Here's how the part is built. I have some questions about the finished solid (model axes, mm). A direction names the side the tool comes from. Round coordinates to 2 decimals unless told otherwise and drop trailing zeros. Loops run counter-clockwise (first coordinate to the right, second up) from the corner with the lowest first, then second, coordinate; pieces in that order, holes last. Notation, with made-up numbers: (26, 33) - (53, 33) arc R10 ccw to (53, 45) - close; hole circle Ø2 at (-8.5, 12.5). An arc over 180 degrees is marked (long way). Answer as a JSON object with one key per item and string values. Group by question number.
1) I want a section at A-A, the plane z = 0.75. Give the number of separate pieces and of enclosed holes in the cut face, then the cut area to 3 significant figures.
2) Will these pins go through, and if not, where does the flat tip stop? P1, Ø1.5, axis at x = 6, y = -3.5, coming from the -Z side; P2, Ø6, axis at y = -6.5, z = 1, coming from the +X side; P3, Ø0.9, axis at y = 9.5, z = 3, coming from the -X side.
3) Which directions (+Z, -Z, +X, -X, +Y, -Y) give clear straight access to the entire face, cutting with the end or side of a thin tool? Please do faces 1 (the face through (-8.35, -0.15, 2.41)), 2 (the face through (6, -3, 4.762)), 3 (the face through (-3.19, -14.35, -2.09)).
4) If we mould it in two halves opening along Y, with no side actions, what happens to faces 4 (the face through (12.7, -0.2, 2.4)), 5 (the face through (0.281, -16.68, -4.017)), 6 (the face through (28.5, -0.2, 2.5))? For each: pulls with the +Y half, pulls with the -Y half, needs draft (parallel to the pull), parting line crosses it, or undercut.
5) I want a section at C-C, the plane x = 0. Please give me the cut outline in (y, z), then the cut area to 3 significant figures.
6) If I drill on line 1 along Y through (x, z) = (0, -1.45); line 2 along Y through (x, z) = (0, 2.6); line 3 along X through (y, z) = (8.5, 4.5), over which ranges is the centre line in solid material (lowest first)? Write a range as [from, to].
from build123d import *

# Parameters (mm, degrees)
F3_DEPTH      = 12.5
F5_DEPTH      = 25
F6_R          = 5
F6_2_R        = 5
F7_F1_R       = 1
F7_F2_R       = 1
F7_F3_R       = 1
F7_F4_R       = 1
F7_F5_R       = 1
F7_F6_R       = 1
F7_F7_R       = 1
F7_F8_R       = 1
F7_2_T1_DEPTH = 4.7461491674
F7_2_T3_DEPTH = 6.508829184
F8_R          = 5
F9_R          = 2
F10_R         = 1
F11_R         = 0.5
F12_R         = 0.99999
F13_R         = 0.5


# Not quite as in the source:
# - a fillet or chamfer that OpenCascade refuses, or shapes differently, is made with other operations: its cross-section is extruded or revolved along the edge and cut away or added
# - a fillet or chamfer is up to 0.001 mm smaller than in the source, because OpenCascade refuses the exact size


with BuildPart() as f1:
    # F0 (on Front) → F1 (revolve)
    with BuildSketch(Plane.XZ):
        Polygon((6.35, 4.7625), (6.35, 0), (12.7, 0), (14.7, 0), (14.7, -1.5), (14.7, -4.61875), (24.5, -4.61875), (28.5, -4.61875), (28.5, 2.38125), (28.5, 9.38125), (24.5, 9.38125), (14.7, 9.38125), (14.7, 6.2625), (14.7, 4.7625), (12.7, 4.7625), align=None)
    revolve(axis=Axis((0, 0, 2.38125), (0, 0, 1)))

    # F2 (on Top) → F3 (cut, symmetric)
    with BuildSketch(Plane.XY):
        Polygon((43.4596711934, -17.25), (17.25, -17.25), (-17.25, -17.25), (-37.0058989125, -17.25), (-37.0058989125, -42.7323755096), (43.4596711934, -42.7323755096), align=None)
        Polygon((-17.25, 17.25), (17.25, 17.25), (41.6040706777, 17.25), (41.6040706777, 42.1191624585), (-37.1745894389, 42.1191624585), (-37.1745894389, 17.25), align=None)
    extrude(amount=F3_DEPTH, both=True, mode=Mode.SUBTRACT)


with BuildPart() as f1b:
    # F0 (on Front) → F1, piece 2 (revolve)
    with BuildSketch(Plane.XZ):
        with BuildLine():
            Line((13.7, -0.7476008326), (12.7, -0.7476008326))
            Line((12.7, -0.7476008326), (0, -0.7476008326))
            Line((0, -0.7476008326), (0, -3.9319758326))
            ThreePointArc((0, -3.9319758326), (4.3942490964, -4.3344919718), (8.6518969432, -5.49375))
            Line((8.6518969432, -5.49375), (10.5085438117, -5.49375))
            Line((10.5085438117, -5.49375), (13.7, -5.49375))
            Line((13.7, -5.49375), (13.7, -1.5))
            Line((13.7, -1.5), (13.7, -0.7476008326))
        make_face()
    revolve(axis=Axis((0, 0, 2.38125), (0, 0, 1)))


with BuildPart() as f1c:
    # F0 (on Front) → F1, piece 3 (revolve)
    with BuildSketch(Plane.XZ):
        with BuildLine():
            Line((0, 8.6944758326), (0, 6.2577016652))
            Line((0, 6.2577016652), (0, 5.5101008326))
            Line((0, 5.5101008326), (12.7, 5.5101008326))
            Line((12.7, 5.5101008326), (13.7, 5.5101008326))
            Line((13.7, 5.5101008326), (13.7, 6.2625))
            Line((13.7, 6.2625), (13.7, 10.25625))
            Line((13.7, 10.25625), (10.5085438117, 10.25625))
            Line((10.5085438117, 10.25625), (8.6518969432, 10.25625))
            ThreePointArc((8.6518969432, 10.25625), (4.3942490964, 9.0969919718), (0, 8.6944758326))
        make_face()
    revolve(axis=Axis((0, 0, 2.38125), (0, 0, 1)))

    # F10
    f10_edges = [f1c.edges().sort_by_distance(p)[0] for p in [
        (-13.7, 0, 10.25625),
    ]]
    fillet(f10_edges, radius=F10_R)


with BuildPart() as f5_tool:
    # F4 (on face) → F5 (new body)
    with BuildSketch(Plane.XY.offset(4.7625)):
        with BuildLine():
            ThreePointArc((-6.4411438468, 10.9453947368), (-12.7, 0), (-6.4411438468, -10.9453947368))
            Line((-6.4411438468, -10.9453947368), (-2, -10.9453947368))
            Line((-2, -10.9453947368), (-2, -8.1069414701))
            ThreePointArc((-2, -8.1069414701), (-8.35, 0), (-2, 8.1069414701))
            Line((-2, 8.1069414701), (-2, 10.9453947368))
            Line((-2, 10.9453947368), (-6.4411438468, 10.9453947368))
        make_face()
        with BuildLine():
            Line((2, -10.9453947368), (6.4411438468, -10.9453947368))
            ThreePointArc((6.4411438468, -10.9453947368), (12.7, 0), (6.4411438468, 10.9453947368))
            Line((6.4411438468, 10.9453947368), (2, 10.9453947368))
            Line((2, 10.9453947368), (2, 8.1069414701))
            ThreePointArc((2, 8.1069414701), (8.35, 0), (2, -8.1069414701))
            Line((2, -8.1069414701), (2, -10.9453947368))
        make_face()
    extrude(amount=-F5_DEPTH)


with BuildPart() as f1_1:
    add(f1.part)

    # F5: cut by f5_tool
    add(f5_tool.part, mode=Mode.SUBTRACT)

    # F6
    f6_edges = [f1_1.edges().sort_by_distance(p)[0] for p in [
        (6.441144, 10.945395, 2.38125),
        (-6.441144, 10.945395, 2.38125),
        (-6.441144, -10.945395, 2.38125),
        (6.441144, -10.945395, 2.38125),
    ]]
    fillet(f6_edges, radius=F6_R)

    # F7: fillet of radius 1 on 8 edges, made by hand

    # F7_f1
    f7_f1_edges = [f1_1.edges().sort_by_distance(p)[0] for p in [
        (-2, 10.9453947368, 2.38125),
    ]]
    fillet(f7_f1_edges, radius=F7_F1_R)

    # F7_f2
    f7_f2_edges = [f1_1.edges().sort_by_distance(p)[0] for p in [
        (-2, 8.1069414701, 2.38125),
    ]]
    fillet(f7_f2_edges, radius=F7_F2_R)

    # F7_f3
    f7_f3_edges = [f1_1.edges().sort_by_distance(p)[0] for p in [
        (-2, -8.1069414701, 2.38125),
    ]]
    fillet(f7_f3_edges, radius=F7_F3_R)

    # F7_f4
    f7_f4_edges = [f1_1.edges().sort_by_distance(p)[0] for p in [
        (-2, -10.9453947368, 2.38125),
    ]]
    fillet(f7_f4_edges, radius=F7_F4_R)

    # F7_f5
    f7_f5_edges = [f1_1.edges().sort_by_distance(p)[0] for p in [
        (2, -10.9453947368, 2.38125),
    ]]
    fillet(f7_f5_edges, radius=F7_F5_R)

    # F7_f6
    f7_f6_edges = [f1_1.edges().sort_by_distance(p)[0] for p in [
        (2, -8.1069414701, 2.38125),
    ]]
    fillet(f7_f6_edges, radius=F7_F6_R)

    # F7_f7
    f7_f7_edges = [f1_1.edges().sort_by_distance(p)[0] for p in [
        (2, 8.1069414701, 2.38125),
    ]]
    fillet(f7_f7_edges, radius=F7_F7_R)

    # F7_f8
    f7_f8_edges = [f1_1.edges().sort_by_distance(p)[0] for p in [
        (2, 10.9453947368, 2.38125),
    ]]
    fillet(f7_f8_edges, radius=F7_F8_R)

    # F8
    f8_edges = [f1_1.edges().sort_by_distance(p)[0] for p in [
        (-22.686725, -17.25, 2.38125),
        (22.686725, -17.25, 2.38125),
        (-22.686725, 17.25, 2.38125),
        (22.686725, 17.25, 2.38125),
    ]]
    fillet(f8_edges, radius=F8_R)

    # F9
    f9_edges = [f1_1.edges().sort_by_distance(p)[0] for p in [
        (0, 17.25, 9.38125),
        (0, 17.25, -4.61875),
    ]]
    fillet(f9_edges, radius=F9_R)

    # F11
    f11_edges = [f1_1.edges().sort_by_distance(p)[0] for p in [
        (-14.7, 0, 9.38125),
    ]]
    fillet(f11_edges, radius=F11_R)

    # F13
    f13_edges = [f1_1.edges().sort_by_distance(p)[0] for p in [
        (-14.7, 0, -4.61875),
    ]]
    fillet(f13_edges, radius=F13_R)


with BuildPart() as f1b_1:
    add(f1b.part)

    # F5: cut by f5_tool
    add(f5_tool.part, mode=Mode.SUBTRACT)

    # F6#2
    f6_2_edges = [f1b_1.edges().sort_by_distance(p)[0] for p in [
        (6.441144, 10.945395, -3.120675),
        (-6.441144, 10.945395, -3.120675),
        (-6.441144, -10.945395, -3.120675),
        (6.441144, -10.945395, -3.120675),
    ]]
    fillet(f6_2_edges, radius=F6_2_R)

    # F7#2: fillet of radius 1 on 8 edges, made by hand

    # F7_2_s2 → F7_2_t1 (join)
    with BuildSketch(Plane.XY.offset(-5.49375)):
        with BuildLine():
            ThreePointArc((-3, 10.9453947368), (-2.2928932188, 10.652501518), (-2, 9.9453947368))
            Line((-2, 9.9453947368), (-1.98, 9.9453947368))
            Line((-1.98, 9.9453947368), (-1.98, 10.9653947368))
            Line((-1.98, 10.9653947368), (-3, 10.9653947368))
            Line((-3, 10.9653947368), (-3, 10.9453947368))
        make_face()
        with BuildLine():
            ThreePointArc((3, -10.9453947368), (2.2928932188, -10.652501518), (2, -9.9453947368))
            Line((2, -9.9453947368), (1.98, -9.9453947368))
            Line((1.98, -9.9453947368), (1.98, -10.9653947368))
            Line((1.98, -10.9653947368), (3, -10.9653947368))
            Line((3, -10.9653947368), (3, -10.9453947368))
        make_face()
        with BuildLine():
            ThreePointArc((2, 9.9453947368), (2.2928932188, 10.652501518), (3, 10.9453947368))
            Line((3, 10.9453947368), (3, 10.9653947368))
            Line((3, 10.9653947368), (1.98, 10.9653947368))
            Line((1.98, 10.9653947368), (1.98, 9.9453947368))
            Line((1.98, 9.9453947368), (2, 9.9453947368))
        make_face()
        with BuildLine():
            ThreePointArc((-2, -9.9453947368), (-2.2928932188, -10.652501518), (-3, -10.9453947368))
            Line((-3, -10.9453947368), (-3, -10.9653947368))
            Line((-3, -10.9653947368), (-1.98, -10.9653947368))
            Line((-1.98, -10.9653947368), (-1.98, -9.9453947368))
            Line((-1.98, -9.9453947368), (-2, -9.9453947368))
        make_face()
    extrude(amount=F7_2_T1_DEPTH)

    # F7_2_s4 → F7_2_t3 (join)
    with BuildSketch(Plane.XY.offset(-7.2564300165)):
        with BuildLine():
            ThreePointArc((2.679144385, 7.908519796), (2.1873329049, 8.2729196832), (2, 8.8556479153))
            Line((2, 8.8556479153), (1.98, 8.8556479153))
            Line((1.98, 8.8556479153), (1.98, 8.1069414701))
            Line((1.98, 8.1069414701), (1.9952095808, 8.0875236462))
            ThreePointArc((1.9952095808, 8.0875236462), (2.3360659907, 7.9957298408), (2.6727272727, 7.8895772336))
            Line((2.6727272727, 7.8895772336), (2.679144385, 7.908519796))
        make_face()
        with BuildLine():
            ThreePointArc((-2, 8.8556479153), (-2.1873329049, 8.2729196832), (-2.679144385, 7.908519796))
            Line((-2.679144385, 7.908519796), (-2.6727272727, 7.8895772336))
            ThreePointArc((-2.6727272727, 7.8895772336), (-2.3360659907, 7.9957298408), (-1.9952095808, 8.0875236462))
            Line((-1.9952095808, 8.0875236462), (-1.98, 8.1069414701))
            Line((-1.98, 8.1069414701), (-1.98, 8.8556479153))
            Line((-1.98, 8.8556479153), (-2, 8.8556479153))
        make_face()
        with BuildLine():
            ThreePointArc((2, -8.8556479153), (2.1873329049, -8.2729196832), (2.679144385, -7.908519796))
            Line((2.679144385, -7.908519796), (2.6727272727, -7.8895772336))
            ThreePointArc((2.6727272727, -7.8895772336), (2.3360659907, -7.9957298408), (1.9952095808, -8.0875236462))
            Line((1.9952095808, -8.0875236462), (1.98, -8.1069414701))
            Line((1.98, -8.1069414701), (1.98, -8.8556479153))
            Line((1.98, -8.8556479153), (2, -8.8556479153))
        make_face()
        with BuildLine():
            ThreePointArc((-2.679144385, -7.908519796), (-2.1873329049, -8.2729196832), (-2, -8.8556479153))
            Line((-2, -8.8556479153), (-1.98, -8.8556479153))
            Line((-1.98, -8.8556479153), (-1.98, -8.1069414701))
            Line((-1.98, -8.1069414701), (-1.9952095808, -8.0875236462))
            ThreePointArc((-1.9952095808, -8.0875236462), (-2.3360659907, -7.9957298408), (-2.6727272727, -7.8895772336))
            Line((-2.6727272727, -7.8895772336), (-2.679144385, -7.908519796))
        make_face()
    extrude(amount=F7_2_T3_DEPTH)

    # F12 (radius 1 in the source; OpenCascade refuses exactly that, so slightly less here)
    f12_edges = [f1b_1.edges().sort_by_distance(p)[0] for p in [
        (-13.7, 0, -5.49375),
    ]]
    fillet(f12_edges, radius=F12_R)


solid = f1_1.part
Outcome:
{
 "1": {"separate pieces": "1", "enclosed holes": "3", "area": "1,470 mm^2"},
 "2": {"P1": "z = 0", "P2": "x = 28.28", "P3": "x = -27.02"},
 "3": {"face 1": "+Z, -Z", "face 2": "+Z", "face 3": "-Z"},
 "4": {"face 4": "undercut", "face 5": "pulls with the -Y half", "face 6": "parting line crosses it"},
 "5": {"outline": "(-17.25, -2.62) arc R2 ccw to (-15.25, -4.62) - (-15.2, -4.62) arc R0.5 ccw to (-14.7, -4.12) - (-14.7, 0) - (-6.35, 0) - (-6.35, 4.76) - (-14.7, 4.76) - (-14.7, 8.88) arc R0.5 ccw to (-15.2, 9.38) - (-15.25, 9.38) arc R2 ccw to (-17.25, 7.38) - close; (6.35, 0) - (14.7, 0) - (14.7, -4.12) arc R0.5 ccw to (15.2, -4.62) - (15.25, -4.62) arc R2 ccw to (17.25, -2.62) - (17.25, 7.38) arc R2 ccw to (15.25, 9.38) - (15.2, 9.38) arc R0.5 ccw to (14.7, 8.88) - (14.7, 4.76) - (6.35, 4.76) - close", "area": "147 mm^2"},
 "6": {"line 1": "[-17.25, -14.7], [14.7, 17.25]", "line 2": "[-17.25, -6.35], [6.35, 17.25]", "line 3": "[-27.2, -9.44], [-2.07, 2.07], [9.44, 27.2]"}
}
